Geometry: final body of the model. Coordinates: model frame, mm. Round coordinates to 2 decimals unless told otherwise and drop trailing zeros. Order: outer loops, then holes, each group sorted by start corner. A loop starts at its lowest first (then second) coordinate and runs counter-clockwise, first axis right, second up. Notation, with made-up numbers: (8.5, -21.75) -> (29.5, -21.75) arc R33 ccw to (29.5, 9.25) -> close; hole circle Ø9 at (80.5, -29). An arc over 180 degrees is marked (long way). Put each result on its own line as item: value.
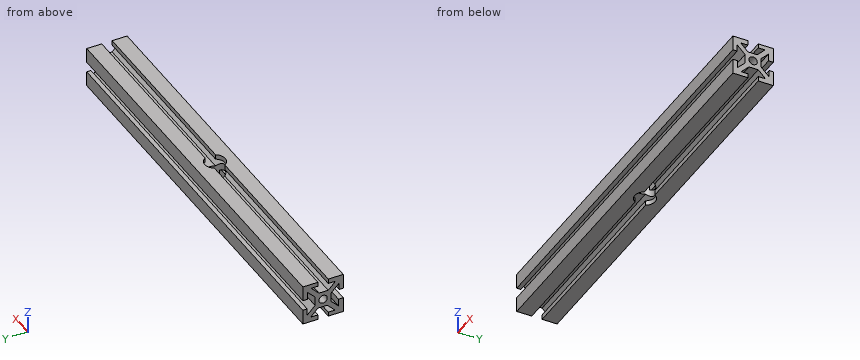
```python
from build123d import *

# Parameters (mm, degrees)
SKETCH1_W           = 10
SKETCH1_H           = 10
SKETCH1_R           = 2.605
BOSS_EXTRUDE1_DEPTH = 254
CIRPATTERN1_COUNT   = 4
SKETCH2_R           = 6.35
CUT_EXTRUDE1_DEPTH  = 30


with BuildPart() as part:
    # Sketch1 → Boss-Extrude1 (new body)
    with BuildSketch(Plane(origin=(0, 0, 0), x_dir=(0, 0, -1), z_dir=(1, 0, 0))):
        Rectangle(SKETCH1_W, SKETCH1_H)
        Circle(SKETCH1_R, mode=Mode.SUBTRACT)
        Polygon((7.474873734, 9.921463197), (2.553410537, 5), (5, 5), (5, 3.203948776), (9.596194078, 7.800142853), align=None)
        Polygon((9.596194078, 3.24), (12.596194078, 3.24), (12.596194078, 12.596194078), (3.24, 12.596194078), (3.24, 9.921463197), (7.474873734, 9.921463197), (9.596194078, 7.800142853), align=None)
    boss_extrude1 = extrude(amount=BOSS_EXTRUDE1_DEPTH)

    # CirPattern1: Boss-Extrude1 ×4 about axis
    cirpattern1_axis = Axis((0, 0, 0), (1, 0, 0))
    for i in range(1, CIRPATTERN1_COUNT):
        add(boss_extrude1.rotate(cirpattern1_axis, i * 360 / CIRPATTERN1_COUNT))

    # Sketch2 → Cut-Extrude1 (cut)
    with BuildSketch(Plane.XY.offset(12.596194078)):
        with Locations((127, 0)):
            Circle(SKETCH2_R)
    extrude(amount=-CUT_EXTRUDE1_DEPTH, mode=Mode.SUBTRACT)


solid = part.part
```
1. Cut plane C-C on x = 127. State how many separate pieces and enclosed holes the cut face has, and give its area (3 significant figures).
Ans:
separate pieces: 4
enclosed holes: 0
area: 194 mm²
2. Material intervals for probe 1 along Y at (x, z) = (144.5, -10.25); probe 2 along Z at (x, y) = (165.5, 0) (3 decimals), sorted ascending.
Ans:
probe 1: -12.6 to -3.24, 3.24 to 12.6
probe 2: -5 to -2.605, 2.605 to 5
3. Cut plane B-B on z = 0. Return loops of the section in (x, y) (3 decimals), and give its area (3 significant figures).
Ans:
outline: (0, -5) -> (123.086, -5) arc R6.35 cw to (121.209, -2.605) -> (0, -2.605) -> close; (0, 2.605) -> (121.209, 2.605) arc R6.35 cw to (123.086, 5) -> (0, 5) -> close; (130.914, -5) -> (254, -5) -> (254, -2.605) -> (132.791, -2.605) arc R6.35 cw to start; (130.914, 5) arc R6.35 cw to (132.791, 2.605) -> (254, 2.605) -> (254, 5) -> close
area: 1,170 mm²
4. Cut plane A-A on y = 0. Return loops of the section in (x, z) (3 decimals).
Ans:
outline: (0, -5) -> (120.65, -5) -> (120.65, -2.605) -> (0, -2.605) -> close; (0, 2.605) -> (120.65, 2.605) -> (120.65, 5) -> (0, 5) -> close; (133.35, -5) -> (254, -5) -> (254, -2.605) -> (133.35, -2.605) -> close; (133.35, 2.605) -> (254, 2.605) -> (254, 5) -> (133.35, 5) -> close
5. Contact query for flat-ended pins moving along their axis: P1, Ø2, axis at x = 44.5, z = 0, coming from the +Y side; P2, Ø3, axis at x = 162.5, z = -1.5, coming from the -Y side. Output: stop coordinate, or through.
Ans:
P1: y = 5
P2: y = -5
